Geometry: final body of the model. Coordinates: model frame, mm. Round coordinates to 2 decimals unless told otherwise and drop trailing zeros. Write each loop counter-clockwise with the first axis right and the second up, starting at its lowest first coordinate (ties: lowest second). Pieces come first, ordered by that corner, then holes. Notation, with made-up numbers: (85.5, 36.5) - (101.5, 36.5) arc R20 cw to (101.5, 42.5) - close; hole circle Ø10 at (80.25, 28). An arc over 180 degrees is marked (long way). Use a Markdown table: item, result. Add a question column.
```python
from build123d import *

# Parameters (mm, degrees)
F0_W     = 39.36
F0_H     = 8.88
F0_R     = 1.17
F1_DEPTH = 5


with BuildPart() as f1:
    # F0 (on Front) → F1 (new body)
    with BuildSketch(Plane.XZ):
        Rectangle(F0_W, F0_H)
        with Locations((-16.51, -1.27)):
            Circle(F0_R, mode=Mode.SUBTRACT)
        with Locations((-13.97, -1.27)):
            Circle(F0_R, mode=Mode.SUBTRACT)
        with Locations((-11.43, -1.27)):
            Circle(F0_R, mode=Mode.SUBTRACT)
        with Locations((-8.89, -1.27)):
            Circle(F0_R, mode=Mode.SUBTRACT)
        with Locations((-6.35, -1.27)):
            Circle(F0_R, mode=Mode.SUBTRACT)
        with Locations((-3.81, -1.27)):
            Circle(F0_R, mode=Mode.SUBTRACT)
        with Locations((-1.27, -1.27)):
            Circle(F0_R, mode=Mode.SUBTRACT)
        with Locations((1.27, -1.27)):
            Circle(F0_R, mode=Mode.SUBTRACT)
        with Locations((3.81, -1.27)):
            Circle(F0_R, mode=Mode.SUBTRACT)
        with Locations((6.35, -1.27)):
            Circle(F0_R, mode=Mode.SUBTRACT)
        with Locations((8.89, -1.27)):
            Circle(F0_R, mode=Mode.SUBTRACT)
        with Locations((11.43, -1.27)):
            Circle(F0_R, mode=Mode.SUBTRACT)
        with Locations((13.97, -1.27)):
            Circle(F0_R, mode=Mode.SUBTRACT)
        with Locations((16.51, -1.27)):
            Circle(F0_R, mode=Mode.SUBTRACT)
        with Locations((-16.51, 1.27)):
            Circle(F0_R, mode=Mode.SUBTRACT)
        with Locations((-13.97, 1.27)):
            Circle(F0_R, mode=Mode.SUBTRACT)
        with Locations((-11.43, 1.27)):
            Circle(F0_R, mode=Mode.SUBTRACT)
        with Locations((-8.89, 1.27)):
            Circle(F0_R, mode=Mode.SUBTRACT)
        with Locations((-6.35, 1.27)):
            Circle(F0_R, mode=Mode.SUBTRACT)
        with Locations((-3.81, 1.27)):
            Circle(F0_R, mode=Mode.SUBTRACT)
        with Locations((-1.27, 1.27)):
            Circle(F0_R, mode=Mode.SUBTRACT)
        with Locations((1.27, 1.27)):
            Circle(F0_R, mode=Mode.SUBTRACT)
        with Locations((3.81, 1.27)):
            Circle(F0_R, mode=Mode.SUBTRACT)
        with Locations((6.35, 1.27)):
            Circle(F0_R, mode=Mode.SUBTRACT)
        with Locations((8.89, 1.27)):
            Circle(F0_R, mode=Mode.SUBTRACT)
        with Locations((11.43, 1.27)):
            Circle(F0_R, mode=Mode.SUBTRACT)
        with Locations((13.97, 1.27)):
            Circle(F0_R, mode=Mode.SUBTRACT)
        with Locations((16.51, 1.27)):
            Circle(F0_R, mode=Mode.SUBTRACT)
    extrude(amount=F1_DEPTH)


solid = f1.part
```
1) Material intervals for L1, parallel to Z at x = 1.27, y = -1.05; L2, parallel to Z at x = 13, y = -4.35, sorted ascending. Write a range as from..to.
2) Draft query along Z for faces 1 (the cylindrical face through (-10.06, -2.46, -1.22)), 2 (the flat face through (-19.68, -2, 0)). Return one class per face: released by +Z, released by -Z, zero draft, split by the parting line, or undercut.
3) Section A-A, the plane x = -8.89. Return the cut outline in (y, z).
4) Section C-C, the plane x = -13.5. Return the cut outline in (y, z).
5) Section B-B, the plane y = -1.1. State how many separate pieces and enclosed holes the cut face has, then the cut area to 3 significant figures.
Output values:
| question | item | result |
|---|---|---|
| 1 | L1 | z = -4.44..-2.44, -0.1..0.1, 2.44..4.44 |
| 1 | L2 | z = -4.44..-1.92, -0.62..0.62, 1.92..4.44 |
| 2 | face 1 | undercut |
| 2 | face 2 | zero draft |
| 3 | outline | (-5, -4.44) - (0, -4.44) - (0, -2.44) - (-5, -2.44) - close; (-5, -0.1) - (0, -0.1) - (0, 0.1) - (-5, 0.1) - close; (-5, 2.44) - (0, 2.44) - (0, 4.44) - (-5, 4.44) - close |
| 4 | outline | (-5, -4.44) - (0, -4.44) - (0, -2.34) - (-5, -2.34) - close; (-5, -0.2) - (0, -0.2) - (0, 0.2) - (-5, 0.2) - close; (-5, 2.34) - (0, 2.34) - (0, 4.44) - (-5, 4.44) - close |
| 5 | separate pieces | 1 |
| 5 | enclosed holes | 28 |
| 5 | area | 229 mm^2 |
